Autodesk Inventor part; units mm, degrees
ref_plane "YZ Plane" through (0, 0, 0) normal (1, 0, 0) x (0, 1, 0)
ref_plane "XZ Plane" through (0, 0, 0) normal (0, 1, 0) x (-1, 0, 0)
ref_plane "XY Plane" through (0, 0, 0) normal (0, 0, 1) x (1, 0, 0)
sketch "Sketch2" plane through (0, 0, 0) normal (0, 0, 1) x (1, 0, 0)
  line L0 (13.0302, 41.5925) -> (13.0302, -41.5925)
  line L1 (13.0302, -41.5925) -> (-13.0302, -41.5925)
  arc A0 (13.0302, 41.5925) -> (-13.0302, -41.5925) centre (53.0449, -16.618) ccw
  point P0 (0, 0)
  point P1 (13.0302, 0)
  point P2 (0, -41.5925)
  dimension "d6" = 26.0604
  dimension "d32" = 70.6374
  dimension "d33" = 83.185
extrude "Extrusion1" add sketch "Sketch2" along normal blind 6
fillet "Fillet2" radius 7.8 1 edges at (-13.0302, -41.5925, 3)
fillet "Fillet3" radius 4.33 1 edges at (13.0302, -41.5925, 3)
sketch "Sketch6" plane through (0, 0, 6) normal (0, 0, 1) x (1, 0, 0)
  line L0 (13.0302, -37.2625) -> (13.0302, 41.5925)
  arc A0 (8.7002, -41.5925) -> (13.0302, -37.2625) centre (8.7002, -37.2625) ccw
  line L1 (13.0302, -37.2625) -> (13.0302, 41.5925)
  arc A1 (13.0302, 41.5925) -> (-14.9029, -35.9244) centre (53.0449, -16.618) ccw
  arc A2 (-14.9029, -35.9244) -> (-7.3999, -41.5925) centre (-7.3999, -33.7925) ccw
  line L2 (-7.3999, -41.5925) -> (8.7002, -41.5925)
  arc A3 (4.2419, -1.0136) -> (13.0302, -26.6511) centre (10.6426, -13.1445) ccw
  line L3 (13.0302, 0.3621) -> (13.0302, -26.6511)
  arc A4 (13.0302, 23.8159) -> (4.2419, -1.0136) centre (13.0302, 9.8459) ccw
  line L4 (13.0302, 0.3621) -> (13.0302, -4.1241)
  line L5 (13.0302, 0.3621) -> (13.0302, 23.8159)
  point P0 (0, 0)
  dimension "d37" = 2.3876
  dimension "d38" = 13.716
  dimension "d39" = 14.732
  dimension "d41" = 50.8
  dimension "d42" = 13.97
extrude "Extrusion4" cut sketch "Sketch6" against normal through all contours A3 A4 L0
sketch "Sketch7" plane through (0, 0, 6) normal (0, 0, 1) x (1, 0, 0)
  arc A0 (13.0302, 23.8159) -> (4.2419, -1.0136) centre (13.0302, 9.8459) ccw
  line L0 (13.0302, 23.8159) -> (13.0302, 41.5925)
  arc A1 (13.0302, 41.5925) -> (-14.9029, -35.9244) centre (53.0449, -16.618) ccw
  arc A2 (-14.9029, -35.9244) -> (-7.3999, -41.5925) centre (-7.3999, -33.7925) ccw
  line L1 (-7.3999, -41.5925) -> (8.7002, -41.5925)
  arc A3 (8.7002, -41.5925) -> (13.0302, -37.2625) centre (8.7002, -37.2625) ccw
  line L2 (13.0302, -37.2625) -> (13.0302, -26.6511)
  arc A4 (4.2419, -1.0136) -> (13.0302, -26.6511) centre (10.6426, -13.1445) ccw
  line L3 (13.0302, 23.8159) -> (13.0302, 41.5925)
  line L4 (13.0302, 23.8159) -> (17.2669, 23.8159) construction
  arc A5 (13.0302, 36.5159) -> (13.0302, 26.3559) centre (13.0302, 31.4359) ccw
  line L5 (13.0302, 36.5159) -> (13.0302, 26.3559)
  point P0 (0, 0)
  dimension "d46" = 10.16
  dimension "d47" = 2.54
extrude "Extrusion5" cut sketch "Sketch7" against normal through all contours A5 L0
sketch "Sketch8" plane through (0, 0, 6) normal (0, 0, 1) x (1, 0, 0)
  arc A0 (13.0302, 36.5159) -> (13.0302, 26.3559) centre (13.0302, 31.4359) ccw
  line L0 (13.0302, 36.5159) -> (13.0302, 41.5925)
  arc A1 (13.0302, 41.5925) -> (-14.9029, -35.9244) centre (53.0449, -16.618) ccw
  arc A2 (-14.9029, -35.9244) -> (-7.3999, -41.5925) centre (-7.3999, -33.7925) ccw
  line L1 (-7.3999, -41.5925) -> (8.7002, -41.5925)
  arc A3 (8.7002, -41.5925) -> (13.0302, -37.2625) centre (8.7002, -37.2625) ccw
  line L2 (13.0302, -37.2625) -> (13.0302, -26.6511)
  arc A4 (4.2419, -1.0136) -> (13.0302, -26.6511) centre (10.6426, -13.1445) ccw
  arc A5 (13.0302, 23.8159) -> (4.2419, -1.0136) centre (13.0302, 9.8459) ccw
  line L3 (13.0302, 23.8159) -> (13.0302, 26.3559)
  line L4 (13.0302, 39.0559) -> (9.5701, 39.0559)
  arc A6 (13.0302, 41.5925) -> (-14.9029, -35.9244) centre (53.0449, -16.618) ccw
  line L5 (13.0302, 36.5159) -> (13.0302, 41.5925)
  point P0 (0, 0)
  dimension "d50" = 2.54
extrude "Extrusion6" cut sketch "Sketch8" against normal through all contours L4 A1 L0
fillet "Fillet4" radius 5.051 1 edges at (13.0302, -26.6511, 3)
sketch "Sketch9" plane through (0, 0, 6) normal (0, 0, 1) x (1, 0, 0)
  arc A0 (13.0302, -31.7215) -> (8.696, -26.7217) centre (7.9792, -31.7215) ccw
  arc A1 (4.2419, -1.0136) -> (8.696, -26.7217) centre (10.6426, -13.1445) ccw
  arc A2 (13.0302, 23.8159) -> (4.2419, -1.0136) centre (13.0302, 9.8459) ccw
  line L0 (13.0302, 23.8159) -> (13.0302, 26.3559)
  arc A3 (13.0302, 36.5159) -> (13.0302, 26.3559) centre (13.0302, 31.4359) ccw
  arc A4 (9.5701, 39.0559) -> (-14.9029, -35.9244) centre (53.0449, -16.618) ccw
  arc A5 (-14.9029, -35.9244) -> (-7.3999, -41.5925) centre (-7.3999, -33.7925) ccw
  line L1 (-7.3999, -41.5925) -> (8.7002, -41.5925)
  arc A6 (8.7002, -41.5925) -> (13.0302, -37.2625) centre (8.7002, -37.2625) ccw
  line L2 (13.0302, -37.2625) -> (13.0302, -31.7215)
  circle A7 centre (8.9027, -37.465) radius 1.5875
  circle A8 centre (-7.0993, -33.8074) radius 1.8415
  line L3 (13.0302, 36.5159) -> (13.0302, 39.0559)
  line L4 (13.0302, 39.0559) -> (9.5701, 39.0559)
  point P0 (0, 0)
  dimension "d54" = 2.54
  dimension "d55" = 2.54
  dimension "d56" = 3.175
  dimension "d57" = 5.9436
  dimension "d58" = 16.002
  dimension "d59" = 3.683
extrude "Extrusion7" cut sketch "Sketch9" against normal through all contours A7 | A8
properties part number "GripperFingersExtended"
Read the model definition and answer for the solid it produces. Units are mm, in the model's axes. A direction names the side the tool comes from. Round coordinates to 2 decimals unless told otherwise and drop trailing zeros. Write each loop counter-clockwise with the first axis right and the second up, starting at its lowest first coordinate (ties: lowest second). Pieces come first, ordered by that corner, then holes.
Q1. Find section A-A on x = -2. Determine the outline of the cut face in (y, z), and give its area (3 significant figures).
Values:
outline: (-41.59, 0) - (-18.46, 0) - (-18.46, 6) - (-41.59, 6) - close; (-7.83, 0) - (27.65, 0) - (27.65, 6) - (-7.83, 6) - close
area: 352 mm2
Q2. Find section B-B on z = 3. Determine the outline of the cut face in (x, y) (1 decimal), and give its area (3 significant figures).
Values:
outline: (-14.9, -35.9) arc R7.8 ccw to (-7.4, -41.6) - (8.7, -41.6) arc R4.3 ccw to (13, -37.3) - (13, -31.7) arc R5.1 ccw to (8.7, -26.7) arc R13.7 cw to (4.2, -1) arc R14 cw to (13, 23.8) - (13, 26.4) arc R5.1 cw to (13, 36.5) - (13, 39.1) - (9.6, 39.1) arc R70.6 ccw to start; hole circle Ø3.7 at (-7.1, -33.8); hole circle Ø3.2 at (8.9, -37.5)
area: 1,260 mm2
Q3. Find section C-C on y = 10. Determine the outline of the cut face in (x, z).
Values:
outline: (-12.39, 0) - (-0.94, 0) - (-0.94, 6) - (-12.39, 6) - close
Q4. A tool of negligible diameter and unlimited length cuts with its end or side. For faces 4 (the face through (11, 39.056, 3)), 5 (the face through (11.763, -28.375, 2.958)), from which of +Z, -Z, +X, -X, +Y, -Y can it reach the whole face along a straight path? Write none if from no direction.
Values:
face 4: +Z, -Z, +X, -X, +Y
face 5: +Z, -Z, +X
Q5. The mould has two halves that part along Y. Classify faces 1 (the face through (-14.3, 4.7, 3)), 2 (the face through (-0.06, 14.73, 3.04)), 3 (the face through (13.03, 25, 3)): released by +Y, released by -Y, zero draft, split by the parting line, or undercut.
Values:
face 1: split by the parting line
face 2: undercut
face 3: zero draft
Q6. Find section D-D on y = -9. Determine the outline of the cut face in (x, z), and give its area (3 significant figures).
Values:
outline: (-17.18, 0) - (-2.43, 0) - (-2.43, 6) - (-17.18, 6) - close
area: 88.5 mm2
Q7. Flat-ended cylindrical pins translate along their axes: P1, Ø2.5, axis at x = 8.9, y = -37.47, coming from the -Z side; P2, Ø1, axis at y = 2, z = 2, coming from the +X side; P3, Ø3, axis at x = 0.5, z = 1, coming from the +Y side; P4, Ø1, axis at x = 9.5, z = 4, coming from the -Y side. Find the tip coordinate at first contact, or state that the pin passes through.
Values:
P1: passes through
P2: stops at x = 1.83
P3: stops at y = 32.21
P4: stops at y = -41.58
Q8. Straight lines are drawn through the part: line 1 (Y direction, x = 3, z = 5); line 2 (Y direction, x = 5, z = 4.4); line 3 (Y direction, x = 2, z = 4.6). For each, find the intervals that lie inside material, in ascending order.
Values:
line 1: y = -41.59 to -24.53, -1.76 to 0.12, 19.57 to 33.23
line 2: y = -41.59 to -25.65, 21.28 to 35.16
line 3: y = -41.59 to -23.8, -2.49 to 1.27, 18.42 to 32.21
